CAD build for the part. Positions are in the model's coordinates, mm. Coordinates: 2 decimals unless noted, no trailing zeros. Loops run counter-clockwise (first coordinate to the right, second up) from the corner with the lowest first, then second, coordinate; pieces in that order, holes last. Notation, with made-up numbers: (-35, 20) -> (6, 20) arc R16 cw to (6, 30) -> close; hole circle Ø10 at (4.25, -16.5). An arc over 180 degrees is marked (long way). Return JSON: item names as keys, results as strings. Group by question number.
(1) Mould opens along Y. For faces 1 (the face through (-0.129, 5.657, -1.377)), 2 (the face through (-3.2, 2.8, 3.979)), 3 (the face through (0.913, 3.913, -9.035)), 4 (the face through (1.483, -1.987, -1.346)) say: pulls with the +Y half, pulls with the -Y half, needs draft (parallel to the pull), parting line crosses it, or undercut.
(2) Saw through at A-A on z = -1.5. Write the cut outline in (x, y).
(3) Probe L1, parallel to X at y = 4, z = -6.25; L2, parallel to X at y = 5.25, z = -0.75; L3, parallel to Y at x = 0.5, z = 3.5. List the from-to ranges inside material, lowest first.
(4) Flat gauge pins, fed straight in: pin 1 Ø1 at (y, z) = (6.5, -5.5) entering from -X; pin 2 Ø4 at (x, y) = (1, 4.5) entering from -Z; pin 3 Ø5 at (y, z) = (6, -4.5) entering from +X; pin 4 Ø5 at (x, y) = (0, 2.72) entering from +Z. Where does each tip first touch, or does it go through?
Autodesk Inventor part; units mm, degrees
ref_plane "YZ Plane" through (0, 0, 0) normal (1, 0, 0) x (0, 1, 0)
ref_plane "XZ Plane" through (0, 0, 0) normal (0, 1, 0) x (-1, 0, 0)
ref_plane "XY Plane" through (0, 0, 0) normal (0, 0, 1) x (1, 0, 0)
sketch "Эскиз1" plane through (0, 0, 0) normal (1, 0, 0) x (0, 1, 0)
  line L0 (-2.2145, -6.8214) -> (-2.2145, 3.9786)
  arc A0 (-2.2145, -6.8214) -> (0.9855, -10.0214) centre (0.9855, -6.8214) ccw
  line L1 (2.7225, -8.0214) -> (2.7225, 3.9786)
  line L2 (-0.2145, 3.9786) -> (-0.2145, -3.8549)
  line L3 (-0.2145, -3.8549) -> (-0.2145, -6.2214)
  line L4 (-0.2145, -6.2214) -> (-0.2145, -6.5844)
  line L5 (1.5855, -8.0214) -> (1.2225, -8.0214)
  arc A1 (-0.2145, -6.5844) -> (1.2225, -8.0214) centre (1.2225, -6.5844) ccw
  line L6 (2.7225, -8.0214) -> (2.7225, 3.9786)
  line L7 (1.2225, -8.0214) -> (1.2225, -10.0214)
  line L8 (1.2225, -10.0214) -> (0.9855, -10.0214)
  line L9 (-0.2145, 3.9786) -> (-2.2145, 3.9786)
  point P0 (1.2855, -8.0214)
  dimension "d1" = 3.2
  dimension "d3" = 14
  dimension "d9" = 2
  dimension "d14" = 1.437
  dimension "d16" = 1.5
sketch "Эскиз2" plane through (0, 0, 0) normal (1, 0, 0) x (0, 1, 0)
  point P0 (0, 0)
sketch "Эскиз3" plane through (0, 0, 0) normal (1, 0, 0) x (0, 1, 0)
  point P0 (0, 0)
sketch "Эскиз4" plane through (0, 0, 0) normal (1, 0, 0) x (0, 1, 0)
  point P0 (0, 0)
revolve "Вращение1" add sketch "Эскиз1" angle 360 about axis through (0, 2.7225, -8.0214) along (0, 0, 1)
properties part number "Задание номер 12"
Geometry results:
{
 "1": {"face 1": "undercut", "face 2": "needs draft", "face 3": "undercut", "face 4": "parting line crosses it"},
 "2": {"outline": "circle Ø9.87 at (0, 2.72); hole circle Ø5.87 at (0, 2.72)"},
 "3": {"L1": "-4.77 to -2.64, 2.64 to 4.77", "L2": "-4.24 to -1.5, 1.5 to 4.24", "L3": "-2.19 to -0.17, 5.62 to 7.63"},
 "4": {"pin 1": "x = -3.69", "pin 2": "z = -10.02", "pin 3": "x = 4.88", "pin 4": "z = -7.61"}
}
